Geometry: final body of the model. Coordinates: model frame, mm. A direction names the side the tool comes from. Give positions to 0.01 mm unless a question says otherwise; leave off trailing zeros. Loops run counter-clockwise (first coordinate to the right, second up) from the corner with the lowest first, then second, coordinate; pieces in that order, holes last. Notation, with made-up numbers: (-14, 85.5) -> (44, 85.5) arc R21 cw to (44, 92.5) -> close; hole circle Ø7 at (18, 21). An arc over 180 degrees is marked (long way). Answer in a Markdown table with one row per item. Add a question column.
1) Line query: line 1 (Y direction, x = 2.5, z = 0.75); line 2 (Z direction, x = 2.5, y = 2); line 3 (X direction, y = -4.5, z = 15.5). Output: solid intervals per line, ascending. Write a range as from..to.
2) Section query A-A (y = 6). Return the cut outline in (x, z), plus the area to 3 significant figures.
3) Section query C-C (z = 14). Return the cut outline in (x, y), plus the area to 3 significant figures.
4) First-contact query: P1, Ø4.5, axis at x = 4, y = 0, coming from the +Z side; P2, Ø10, axis at x = 5, z = 4.5, coming from the +Y side; P3, Ø1, axis at y = 0.5, z = 4, coming from the -X side. Flat tips, straight axial feed; report the tip coordinate or a pass-through.
5) Draft query along Y for faces 1 (the flat face through (9.5, 0, 14)), 2 (the cylindrical face through (1.31, 0.38, 1.23)), 3 (the flat face through (11, 9, 14)). Return one class per face: +Y half, -Y half, draft (parallel to the pull), parting line (faces both ways), or undercut.
6) Section query B-B (y = 0). Return the cut outline in (x, z).
7) Section query D-D (x = 12.25). Return the cut outline in (y, z).
8) Access query for faces 4 (the cylindrical face through (9.4, 0, 0.8)), 5 (the flat face through (4, 0, 2.5)), 6 (the flat face through (9, -2.75, 4)), 7 (the flat face through (9, 2.75, 4)), 8 (the cylindrical face through (12.493, 5.7, 14.954)). Directions: +Z, -Z, +X, -X, +Y, -Y. A direction counts if a zero-diameter tool reaches every point of the face in a straight line with its end or side. Return the directions, or none.
```python
from build123d import *

# Parameters (mm, degrees)
EXTRUDE_1_DEPTH     = 2.75
SKETCH_2_R          = 1.25
CUT_EXTRUDE_1_DEPTH = 10
FILLET_2_R          = 2.5
SKETCH_4_W          = 6
SKETCH_4_H          = 18
EXTRUDE_2_DEPTH     = 2.5
SKETCH_5_R          = 1
EXTRUDE_3_DEPTH     = 1


with BuildPart() as part:
    # 草图1 → 凸台-拉伸1 (new, symmetric)
    with BuildSketch(Plane(origin=(0, 0, 0), x_dir=(1, 0, 0), z_dir=(0, 1, 0))):
        with BuildLine():
            Line((0, 0), (7, 0))
            ThreePointArc((7, 0), (9.461409331, -0.846991262), (10.880422565, -3.029267947))
            Line((10.880422565, -3.029267947), (11.831813783, -6.832377099))
            ThreePointArc((11.831813783, -6.832377099), (11.957795141, -7.509886755), (12, -8.197716229))
            Line((12, -8.197716229), (12, -17))
            Line((12, -17), (9.5, -17))
            Line((9.5, -17), (9.5, -8.197716229))
            ThreePointArc((9.5, -8.197716229), (9.47654946, -7.815533399), (9.40654968, -7.439084632))
            Line((9.40654968, -7.439084632), (8.455158462, -3.63597548))
            ThreePointArc((8.455158462, -3.63597548), (7.923028499, -2.817621723), (7, -2.5))
            Line((7, -2.5), (0, -2.5))
            Line((0, -2.5), (0, 0))
        make_face()
    extrude(amount=EXTRUDE_1_DEPTH, both=True)

    # 草图2 → 切除-拉伸1 (cut)
    with BuildSketch(Plane(origin=(0, 0, 0), x_dir=(-1, 0, 0), z_dir=(0, 0, -1))):
        with Locations((-2.5, 0)):
            Circle(SKETCH_2_R)
    extrude(amount=-CUT_EXTRUDE_1_DEPTH, mode=Mode.SUBTRACT)

    # 圆角2
    fillet_2_edges = [part.edges().sort_by_distance(p)[0] for p in [
        (0, -2.75, 1.25),
        (0, 2.75, 1.25),
    ]]
    fillet(fillet_2_edges, radius=FILLET_2_R)

    # 草图4 → 凸台-拉伸2 (add)
    with BuildSketch(Plane.ZY.offset(-9.5)):
        with Locations((14, 0)):
            Rectangle(SKETCH_4_W, SKETCH_4_H)
    extrude(amount=-EXTRUDE_2_DEPTH)

    # 草图5 → 凸台-拉伸3 (add)
    with BuildSketch(Plane(origin=(12, 0, 0), x_dir=(0, 0, -1), z_dir=(1, 0, 0))):
        with Locations(Location((-14, 6, 0), (0, 0, 180))):
            Circle(SKETCH_5_R)
    extrude_3 = extrude(amount=EXTRUDE_3_DEPTH)

    # 草图6 → 旋转1 (revolve)
    with BuildSketch(Plane(origin=(0, 0, 14), x_dir=(-1, 0, 0), z_dir=(0, 0, -1))):
        with BuildLine():
            Line((-13, 6), (-16.732050808, 6))
            ThreePointArc((-16.732050808, 6), (-15.249688898, 7.931851653), (-13, 7))
            Line((-13, 7), (-13, 6))
        make_face()
    revolve_1 = revolve(axis=Axis((13, 6, 14), (1, 0, 0)))

    # 镜向1: 凸台-拉伸3, 旋转1 across plane
    add(extrude_3.mirror(Plane.ZX))
    add(revolve_1.mirror(Plane.ZX))


solid = part.part
```
Evaluation:
| question | item | result |
|---|---|---|
| 1 | line 1 | -2.75..-1.25, 1.25..2.75 |
| 1 | line 2 | 0..2.5 |
| 1 | line 3 | 9.5..12 |
| 2 | outline | (9.5, 11) -> (12, 11) -> (12, 13) -> (13, 13) arc R2 ccw (long way) to (13, 15) -> (12, 15) -> (12, 17) -> (9.5, 17) -> close |
| 2 | area | 29.2 mm² |
| 3 | outline | (9.5, -9) -> (12, -9) -> (12, -7) -> (13, -7) arc R2 ccw (long way) to (13, -5) -> (12, -5) -> (12, 5) -> (13, 5) arc R2 ccw (long way) to (13, 7) -> (12, 7) -> (12, 9) -> (9.5, 9) -> close |
| 3 | area | 73.4 mm² |
| 4 | P1 | z = 2.5 |
| 4 | P2 | y = 2.75 |
| 4 | P3 | x = 8.41 |
| 5 | face 1 | draft |
| 5 | face 2 | undercut |
| 5 | face 3 | +Y half |
| 6 | outline | (0, 0) -> (1.25, 0) -> (1.25, 2.5) -> (0, 2.5) -> close; (3.75, 0) -> (7, 0) arc R4 ccw to (10.88, 3.03) -> (11.83, 6.83) arc R5.63 ccw to (12, 8.2) -> (12, 17) -> (9.5, 17) -> (9.5, 8.2) arc R3.13 cw to (9.41, 7.44) -> (8.46, 3.64) arc R1.5 cw to (7, 2.5) -> (3.75, 2.5) -> close |
| 7 | outline | circle Ø2 at (-6, 14); circle Ø2 at (6, 14) |
| 8 | face 4 | -Z, +X, +Y, -Y |
| 8 | face 5 | +Z, -X, +Y, -Y |
| 8 | face 6 | -Z, +X, -X, -Y |
| 8 | face 7 | -Z, +X, -X, +Y |
| 8 | face 8 | none |
